Check sheet for the modelled part. Datum: model origin and axes. Units: mm. Face numbers are marked on the shaded views. A direction names the side the tool comes from. Give positions to 0.01 mm unless a question says otherwise; leave off trailing zeros. Order: outer loops, then holes, each group sorted by start corner. A loop starts at its lowest first (then second) coordinate and runs counter-clockwise, first axis right, second up.
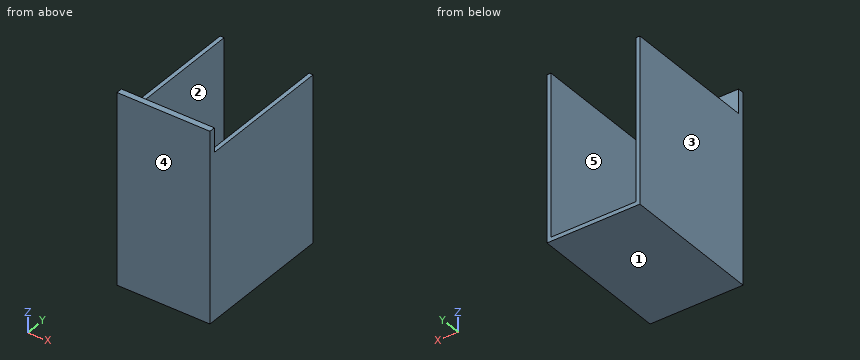
```python
from build123d import *

# Parameters (mm, degrees)
SKETCH1_W           = 292.1
SKETCH1_H           = 596.9
BOSS_EXTRUDE1_DEPTH = 19.05
BOSS_EXTRUDE2_DEPTH = 425.45


with BuildPart() as part:
    # Sketch1 → Boss-Extrude1 (new body)
    with BuildSketch(Plane(origin=(0, 0, 0), x_dir=(1, 0, 0), z_dir=(0, 1, 0))):
        Rectangle(SKETCH1_W, SKETCH1_H)
    extrude(amount=BOSS_EXTRUDE1_DEPTH)

    # Sketch2 → Boss-Extrude2 (add)
    with BuildSketch(Plane(origin=(0, 19.05, 0), x_dir=(1, 0, 0), z_dir=(0, 1, 0))):
        Polygon((-146.05, -222.25), (-146.05, 298.45), (146.05, 298.45), (146.05, -222.25), (133.35, -222.25), (133.35, 285.75), (-133.35, 285.75), (-133.35, -222.25), align=None)
    extrude(amount=BOSS_EXTRUDE2_DEPTH)


solid = part.part
```
(1) Set-up check for the marked faces 1 and 2: record each of +Z, -Z, +X, -X, +Y, -Y from which the full face is reachable in a straight line by a thin tool's end or side.
Response values:
face 1: -Z, +X, -X, +Y, -Y
face 2: +Z, +Y
(2) Gauge pin test, flat ends, axial feed: pin 1 Ø2 at (x, y) = (-74.5, 224) entering from +Z; pin 2 Ø10 at (x, y) = (140, 205.5) entering from +Z. Record the tip position at first contact, or that the pin passes through.
Response values:
pin 1: stops at z = -285.75
pin 2: stops at z = 222.25
(3) Release check for a two-part mould opening along X. For the marked faces 3, 4 and 5 record: released by +X, released by -X, zero draft, split by the parting line, or undercut.
Response values:
face 3: released by -X
face 4: zero draft
face 5: undercut
(4) Cross-section at A-A on x = 13. Enter the section's corners in (y, z), then the cut area to 3 significant figures.
Response values:
outline: (0, -298.45) - (444.5, -298.45) - (444.5, -285.75) - (19.05, -285.75) - (19.05, 298.45) - (0, 298.45) - close
area: 16,800 mm2
(5) Cross-section at C-C on y = 276. Enter the section's corners in (x, z), then the cut area to 3 significant figures.
Response values:
outline: (-146.05, -298.45) - (146.05, -298.45) - (146.05, 222.25) - (133.35, 222.25) - (133.35, -285.75) - (-133.35, -285.75) - (-133.35, 222.25) - (-146.05, 222.25) - close
area: 16,600 mm2
(6) Material ranges on L1, parallel to X at y = 83, z = -53.5; L2, parallel to Z at x = -110, y = 328.5; L3, parallel to Y at x = -65.5, z = -154.5, recorded low to high.
Response values:
L1: x = -146.05 to -133.35, 133.35 to 146.05
L2: z = -298.45 to -285.75
L3: y = 0 to 19.05
(7) Cross-section at B-B on z = -4. Enter the section's corners in (x, y), then the cut area to 3 significant figures.
Response values:
outline: (-146.05, 0) - (146.05, 0) - (146.05, 444.5) - (133.35, 444.5) - (133.35, 19.05) - (-133.35, 19.05) - (-133.35, 444.5) - (-146.05, 444.5) - close
area: 16,400 mm2
